Autodesk Inventor part; units mm, degrees
ref_plane "Work Plane1" through (3.5, 0, 0) normal (0, 0, 1) x (1, 0, 0)
ref_plane "YZ Plane" through (0, 0, 0) normal (1, 0, 0) x (0, 1, 0)
ref_plane "XZ Plane" through (0, 0, 0) normal (0, 1, 0) x (-1, 0, 0)
sketch "Sketch1" plane through (0, 0, 0) normal (0, 0, 1) x (1, 0, 0)
  line L0 (0, 5.2578) -> (0, 2.413)
  line L1 (2.6458, 2.413) -> (19.05, 2.413)
  line L2 (19.05, 2.413) -> (19.05, 0)
  line L3 (19.05, 0) -> (-0.7874, 0)
  line L4 (0, -1.0516) -> (0, 6.3094)
  line L5 (-4.7549, 0) -> (23.0175, 0)
  line L6 (-0.7874, 0) -> (-0.7874, 5.2578)
  line L7 (-0.7874, 5.2578) -> (0, 5.2578)
  line L8 (2.6458, 2.413) -> (0, 2.413)
  line L9 (0, 2.413) -> (0, 2.413)
  dimension "d0" = 19.05
  dimension "d1" = 16.4042
  dimension "d2" = 4.826
  dimension "d8" = 0.7874
  dimension "d9" = 10.5156
  dimension "d15" = 4.826
  dimension "d16" = 2.6458
revolve "Body" add sketch "Sketch1" angle 360 about axis through (19.05, 0, 0) along (-1, 0, 0)
sketch "Sketch2" plane through (0, 0, 0) normal (1, 0, 0) x (0, 0, -1)
  circle A0 centre (0, 0) radius 5.2578
  line L0 (0, 4.5754) -> (3.9624, 2.2877)
  line L1 (3.9624, 2.2877) -> (3.9624, -2.2877)
  line L2 (3.9624, -2.2877) -> (0, -4.5754)
  line L3 (0, -4.5754) -> (-3.9624, -2.2877)
  line L4 (-3.9624, -2.2877) -> (-3.9624, 2.2877)
  line L5 (-3.9624, 2.2877) -> (0, 4.5754)
  circle A1 centre (0, 0) radius 5.2578
  dimension "d10" = 7.9248
extrude "Head" add sketch "Sketch2" against normal blind 3.048 contours L0 L1 L2 L3 L4 L5
sketch "Sketch3" plane through (0, 0, 0) normal (0, 0, 1) x (1, 0, 0)
  line L0 (-3.048, 3.9624) -> (-3.048, 4.5754)
  line L1 (-3.048, 4.5754) -> (-2.6941, 4.5754)
  line L2 (-2.6941, 4.5754) -> (-3.048, 3.9624)
  line L3 (-2.0219, 4.5754) -> (-3.048, 4.5754)
  line L4 (-3.048, 4.5754) -> (-3.048, 2.266)
  line L5 (-0.7874, 4.5754) -> (-3.048, 4.5754)
  line L6 (-3.048, 4.5754) -> (-3.048, 2.2877)
  line L7 (-3.5001, 0) -> (-0.3353, 0)
  dimension "d5" = 30
  dimension "d18" = 7.9248
revolve "Chamfer1" cut sketch "Sketch3" angle 360 about axis through (-10, 0, 0) along (1, 0, 0)
thread "Thread"
chamfer "Chamfer2" distance 0.6492 distance2 0.6492 1 edges at (19.05, -2.413, 0) measured on face at (19.05, -0.4919, 0.3738)
ref_plane "Work Plane1" through (3.5, 0, 0) normal (0, 0, 1) x (1, 0, 0)
equation "\"d10\" = SW"
equation "\"d3\" = KOH"
equation "\"d13\" = GEL"
equation "\"d6\" = -0.5 * SPD + 0.5 * GD"
equation "\"d7\" = -0.5 * SPD + 0.5 * GD"
equation "\"d0\" = NLG"
equation "\"d1\" = GEL"
equation "\"d2\" = GD"
equation "\"d8\" = PHH"
equation "\"d9\" = LADI"
equation "\"d15\" = BDM"
equation "\"d16\" = GAL"
equation "\"d5\" = ANG1"
equation "\"d18\" = SW0"
equation "\"NLG\" = 19.05"
equation "\"GD\" = NND"
equation "\"BDM\" = NND"
equation "\"KOH\" = 3.048"
equation "\"GEL\" = 16.40416"
equation "\"LADI\" = 10.5156"
equation "\"SW\" = 7.9248"
equation "\"PHH\" = 0.7874"
equation "\"SW0\" = 7.9248"
equation "\"SPD\" = GD1"
equation "\"ANG1\" = 30deg"
equation "\"GAL\" = 2.64584"
equation "\"GUL\" = GAL"
equation "\"GD1\" = 3.52753"
equation "\"THREADDIA\" = 4.826"
equation "\"SDH\" = SW"
equation "\"TOA\" = 30deg"
equation "\"RR\" = 0.04826"
equation "\"NND\" = 4.826"
equation "\"SD\" = 0"
equation "\"SD2\" = NND"
equation "\"E0\" = 8.636"
properties part number "ANSI B18.6.3 - 10-24 UNC x 0.75" material "Steel, Mild"
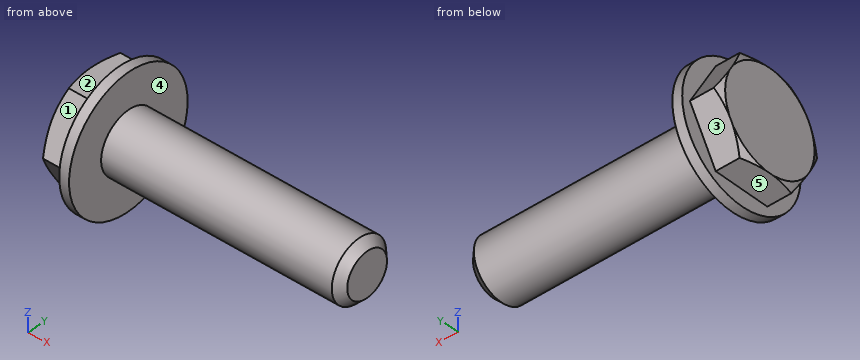
Here's how the part is built. I have some questions about the finished solid (model axes, mm). Face numbers are marked on the shaded views. A direction names the side the tool comes from. Coordinates: 2 decimals unless noted, no trailing zeros. Order: outer loops, then holes, each group sorted by start corner. A loop starts at its lowest first (then second) coordinate and runs counter-clockwise, first axis right, second up. Notation, with made-up numbers: M 73.5,27 L 128.5,27 A19 cw 128.5,39 Z; hole C 59.25,-32.75 d4. An arc over 180 degrees is marked long. Answer as CSV lines item,"result". Start each with the question number.
1. On a 3-axis mill with a long thin cutter (end or side, diameter ignored), from which of +Z, -Z, +X, -X, +Y, -Y can I reach the whole of each face in a straight line? I mean the marked faces 1, 2, 3, 4 and 5. Say none if no direction works.
2. For pin 1 (2 mm diameter, centred on y = -3.5, z = -4, fed in from -X); pin 2 (4 mm diameter, centred on x = 5, y = -1, fed in from -Z); pin 3 (6 mm diameter, centred on x = 0.5, z = 2.5, fed in from -Y); pin 4 (0.7 mm diameter, centred on x = -1.5, y = 0, fed in from +Z), each with a flat end and sliding along its axis, tell me the tip position at first contact or that it passes through.
3. I want a section at A-A, the plane x = 4.5. Write out the boundary of the cut face in (y, z).
4. I need wall thicknesses on line 1 (X direction, y = 4.75, z = -0.75); line 2 (Z direction, x = 4.75, y = 0); line 3 (Z direction, x = -1.5, y = 0.5). Which ranges of each line are inside material? Lowest first, please. Write a range as [from, to].
Recorded:
1,face 1,"+Z, -X, -Y"
1,face 2,"+Z, -X, +Y, -Y"
1,face 3,"-Z, -X, +Y"
1,face 4,"+X"
1,face 5,"-Z, -X, +Y, -Y"
2,pin 1,"stops at x = -0.79"
2,pin 2,"stops at z = -2.41"
2,pin 3,"stops at y = -5.26"
2,pin 4,"stops at z = 3.96"
3,outline,"C 0,0 d4.83"
4,line 1,"x = [-0.79, 0]"
4,line 2,"z = [-2.41, 2.41]"
4,line 3,"z = [-3.96, 3.96]"
